Source: CAD feature listing. Evaluate the final solid. Frame: model axes, mm. A direction names the side the tool comes from. Round coordinates to 2 decimals unless told otherwise and drop trailing zeros. Order: outer loops, then holes, each group sorted by start corner. A loop starts at its lowest first (then second) coordinate and runs counter-clockwise, first axis right, second up. Notation, with made-up numbers: M 33.25,8.5 L 87.25,8.5 A32 cw 87.25,34.5 Z; hole C -27,-34 d9. An arc over 180 degrees is marked long. Use one line per item in the form item = value. Start each with the question number.
Q1. Reachability of faces 1 (the flat face through (-55.079, -13.686, 50.479)), 2 (the flat face through (5, -2.349, 1)), 3 (the flat face through (15.061, 36, 50)), 4 (the flat face through (-48, 24.651, 26)) from +Z, -Z, +X, -X, +Y, -Y: full face, straight path, thin tool, end or side. Return the list, or none.
Q2. Material intervals for probe 1 along Z at (x, y) = (20, 16); probe 2 along Y at (x, z) = (-64, 29), sorted ascending.
Q3. Section D-D (x = -57.5). Return the cut outline in (y, z), plus the area to 3 significant figures.
Q4. Contact query for flat-ended pins moving along their axis: pin 1 (11.5 mm diameter, centred on x = 15.06, y = 17.65, fed in from +Z); pin 2 (14 mm diameter, centred on x = -37, z = 30.5, fed in from -Y); pin 3 (0.9 mm diameter, centred on y = 27, z = 29.5, fed in from +X); pin 4 (2.5 mm diameter, centred on y = 36, z = 2, fed in from +X). Output: stop coordinate, or through.
Q5. Section B-B (y = -13). Return the cut outline in (x, z).
Q6. Section A-A (x = 6). Return the cut outline in (y, z).
Q7. Pull-direction query (Z, two-part tool) for faces 5 (the flat face through (-10.859, 26, 26)), 6 (the flat face through (-35.08, -13.37, 1.48)), 7 (the flat face through (-28, 14, 52)); classes: pulls with the +Z half, pulls with the -Z half, needs draft (parallel to the pull), parting line crosses it, or undercut.
from build123d import *

# Parameters (mm, degrees)
F0_R     = 5
F1_DEPTH = 52
F2_W     = 31.6232873572
F2_H     = 46
F2_W_2   = 27
F2_W_3   = 8.3583824264
F2_W_4   = 10
F3_DEPTH = 116.001
F4_R     = 2.99999
F5_W     = 50
F5_H     = 46
F6_DEPTH = 52.361679775


# Not quite as in the source:
# - a fillet or chamfer is up to 0.001 mm smaller than in the source, because OpenCascade refuses the exact size


with BuildPart() as f1:
    # F0 (on Top) → F1 (new body)
    with BuildSketch(Plane.XY):
        with BuildLine():
            Line((15.0605264698, 33.6507520748), (15.0605264698, 37.6507520748))
            Line((15.0605264698, 37.6507520748), (-84.9394735302, 37.6507520748))
            Line((-84.9394735302, 37.6507520748), (-84.9394735302, -2.3492479252))
            Line((-84.9394735302, -2.3492479252), (-64.9394735302, -24.7099277002))
            Line((-64.9394735302, -24.7099277002), (-44.9394735302, -2.3492479252))
            Line((-44.9394735302, -2.3492479252), (-24.9394735302, -24.7099277002))
            Line((-24.9394735302, -24.7099277002), (-4.9394735302, -2.3492479252))
            Line((-4.9394735302, -2.3492479252), (15.0605264698, -2.3492479252))
            Line((15.0605264698, -2.3492479252), (24.6605264698, 4.8507520748))
            ThreePointArc((24.6605264698, 4.8507520748), (30.2394592386, 22.7103963311), (15.0605264698, 33.6507520748))
        make_face()
        with Locations((15.0605264698, 17.6507520748)):
            Circle(F0_R, mode=Mode.SUBTRACT)
    extrude(amount=F1_DEPTH)

    # F2 (on face) → F3 (cut, through all)
    with BuildSketch(Plane(origin=(-84.9394735302, 0, 0), x_dir=(0, -1, 0), z_dir=(-1, 0, 0))):
        with Locations((18.1608916038, 26)):
            Rectangle(F2_W, F2_H)
        with Locations((-11.1507520748, 26)):
            Rectangle(F2_W_2, F2_H)
        with Locations((-41.829943288, 26)):
            Rectangle(F2_W_3, F2_H)
        with Locations((-32.6507520748, 26)):
            Rectangle(F2_W_4, F2_H)
    extrude(amount=-F3_DEPTH, mode=Mode.SUBTRACT)

    # F4 (radius 3 in the source; OpenCascade refuses exactly that, so slightly less here)
    f4_edges = [f1.edges().sort_by_distance(p)[0] for p in [
        (27.550522, 27.650752, 26),
        (-84.939474, 27.650752, 26),
    ]]
    fillet(f4_edges, radius=F4_R)

    # F5 (on face) → F6 (cut, through all)
    with BuildSketch(Plane(origin=(0, 27.6507520748, 0), x_dir=(-1, 0, 0), z_dir=(0, 1, 0))):
        with Locations((-14.1408709809, 26)):
            Rectangle(F5_W, F5_H)
    extrude(amount=-F6_DEPTH, mode=Mode.SUBTRACT)


solid = f1.part
Results list:
q1.face_1 = +Z, -Z, -Y
q1.face_2 = +Z, -Z, +X, -Y
q1.face_3 = +Z, -Z, +X, +Y
q1.face_4 = +X, -X, -Y
q2.probe_1 = 0 to 3, 49 to 52
q2.probe_2 = 24.65 to 27.65
q3.outline = M -16.39,0 L 37.65,0 L 37.65,3 L 27.65,3 L 27.65,49 L 37.65,49 L 37.65,52 L -16.39,52 L -16.39,49 L 24.65,49 L 24.65,3 L -16.39,3 Z
q3.area = 462 mm2
q4.pin_1 = 52
q4.pin_2 = 24.65
q4.pin_3 = -10.86
q4.pin_4 = 15.06
q5.outline = M -75.41,0 L -54.47,0 L -54.47,3 L -75.41,3 Z; M -75.41,49 L -54.47,49 L -54.47,52 L -75.41,52 Z; M -35.41,0 L -14.47,0 L -14.47,3 L -35.41,3 Z; M -35.41,49 L -14.47,49 L -14.47,52 L -35.41,52 Z
q6.outline = M -2.35,0 L 37.65,0 L 37.65,3 L -2.35,3 Z; M -2.35,49 L 37.65,49 L 37.65,52 L -2.35,52 Z
q7.face_5 = undercut
q7.face_6 = needs draft
q7.face_7 = pulls with the +Z half
